Source: CAD feature listing. Evaluate the final solid. Frame: model axes, mm. Give positions to 0.01 mm unless a question says otherwise; leave off trailing zeros. Write each loop counter-clockwise with the first axis right and the second up, starting at its lowest first coordinate (ties: lowest second). Pieces come first, ordered by that corner, then holes. Notation, with made-up numbers: M 14,46.5 L 29,46.5 A34 ccw 29,80.5 Z; hole C 8,27.25 d4. An arc over 180 degrees is marked long. Answer as a JSON object with one key per item and string values. Group by question number.
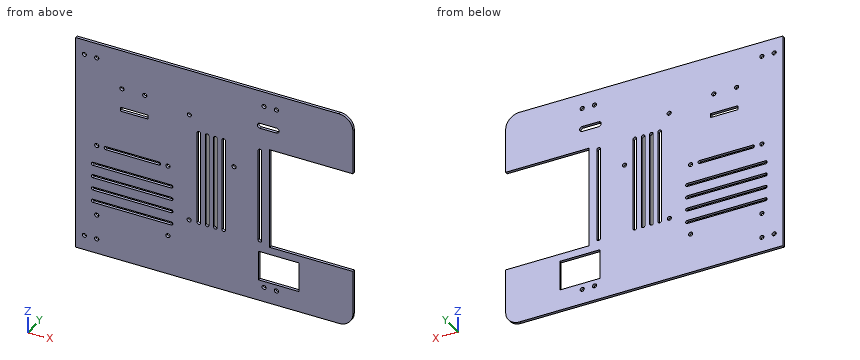
```python
from build123d import *

# Parameters (mm, degrees)
BOSS_EXTRUDE1_DEPTH = 2
SKETCH2_R           = 1.5
SKETCH2_W           = 19.920515559
SKETCH2_H           = 3.018311412
SKETCH2_W_2         = 29
SKETCH2_H_2         = 22
CUT_EXTRUDE1_DEPTH  = 2
FILLET1_R           = 10


with BuildPart() as part:
    # Sketch1 → Boss-Extrude1 (new body)
    with BuildSketch(Plane(origin=(0, 0, 0), x_dir=(1, 0, 0), z_dir=(0, 1, 0))):
        Polygon((62.5, -37.5), (62.5, -80.53), (-137.5, -80.53), (-137.5, 80.53), (62.5, 80.53), (62.5, 37.5), (2.5, 37.5), (2.5, -37.5), align=None)
    extrude(amount=BOSS_EXTRUDE1_DEPTH)

    # Sketch2 → Cut-Extrude1 (cut)
    with BuildSketch(Plane(origin=(0, 2, 0), x_dir=(1, 0, 0), z_dir=(0, 1, 0))):
        with Locations(Location((-131.256523302, -69.515826612, 0), (0, 0, 270))):
            Circle(SKETCH2_R)
        with Locations(Location((7.303150728, -69.515826612, 0), (0, 0, 270))):
            Circle(SKETCH2_R)
        with Locations(Location((-131.256523302, 69.515826612, 0), (0, 0, 90))):
            Circle(SKETCH2_R)
        with Locations(Location((7.303150728, 69.515826612, 0), (0, 0, 90))):
            Circle(SKETCH2_R)
        with Locations(Location((-122.332492344, -69.515826612, 0), (0, 0, 270))):
            Circle(SKETCH2_R)
        with Locations(Location((-1.623456056, -69.515826612, 0), (0, 0, 270))):
            Circle(SKETCH2_R)
        with Locations(Location((-1.623456056, 69.515826612, 0), (0, 0, 270))):
            Circle(SKETCH2_R)
        with Locations(Location((-122.332492344, 69.515826612, 0), (0, 0, 270))):
            Circle(SKETCH2_R)
        with Locations(Location((-23.238563778, -16.512077665, 0), (0, 0, 270))):
            Circle(SKETCH2_R)
        with Locations(Location((-55.491043914, -46.437145858, 0), (0, 0, 270))):
            Circle(SKETCH2_R)
        with Locations(Location((-55.618758711, 34.282977792, 0), (0, 0, 270))):
            Circle(SKETCH2_R)
        with Locations(Location((-70.912492344, 51.192828944, 0), (0, 0, 270))):
            Circle(SKETCH2_R)
        with Locations(Location((-122.332492344, 51.192828944, 0), (0, 0, 270))):
            Circle(SKETCH2_R)
        with Locations(Location((-122.332492344, -2.227171201, 0), (0, 0, 270))):
            Circle(SKETCH2_R)
        with Locations(Location((-70.912492344, -2.227171201, 0), (0, 0, 270))):
            Circle(SKETCH2_R)
        with Locations(Location((-104.14455224, -51.392693568, 0), (0, 0, 270))):
            Circle(SKETCH2_R)
        with Locations(Location((-87.673175627, -51.392693568, 0), (0, 0, 270))):
            Circle(SKETCH2_R)
        with BuildLine():
            Line((-3.265151958, 34.282977792), (-3.265151958, -34.42226179))
            ThreePointArc((-3.265151958, -34.42226179), (-4.562464061, -35.719573893), (-5.859776165, -34.42226179))
            Line((-5.859776165, -34.42226179), (-5.859776165, 34.282977792))
            ThreePointArc((-5.859776165, 34.282977792), (-4.562464061, 35.580289895), (-3.265151958, 34.282977792))
        make_face()
        with BuildLine():
            Line((-29.373558034, 34.282977792), (-29.373558034, -34.42226179))
            ThreePointArc((-29.373558034, -34.42226179), (-30.670870138, -35.719573893), (-31.968182241, -34.42226179))
            Line((-31.968182241, -34.42226179), (-31.968182241, 34.282977792))
            ThreePointArc((-31.968182241, 34.282977792), (-30.670870138, 35.580289895), (-29.373558034, 34.282977792))
        make_face()
        with BuildLine():
            Line((-35.373558034, 34.282977792), (-35.373558034, -34.42226179))
            ThreePointArc((-35.373558034, -34.42226179), (-36.670870138, -35.719573893), (-37.968182241, -34.42226179))
            Line((-37.968182241, -34.42226179), (-37.968182241, 34.282977792))
            ThreePointArc((-37.968182241, 34.282977792), (-36.670870138, 35.580289895), (-35.373558034, 34.282977792))
        make_face()
        with BuildLine():
            Line((-41.373558034, 34.282977792), (-41.373558034, -34.42226179))
            ThreePointArc((-41.373558034, -34.42226179), (-42.670870138, -35.719573893), (-43.968182241, -34.42226179))
            Line((-43.968182241, -34.42226179), (-43.968182241, 34.282977792))
            ThreePointArc((-43.968182241, 34.282977792), (-42.670870138, 35.580289895), (-41.373558034, 34.282977792))
        make_face()
        with BuildLine():
            Line((-47.373558034, 34.282977792), (-47.373558034, -34.42226179))
            ThreePointArc((-47.373558034, -34.42226179), (-48.670870138, -35.719573893), (-49.968182241, -34.42226179))
            Line((-49.968182241, -34.42226179), (-49.968182241, 34.282977792))
            ThreePointArc((-49.968182241, 34.282977792), (-48.670870138, 35.580289895), (-47.373558034, 34.282977792))
        make_face()
        with BuildLine():
            Line((-115.769074494, -1.056435162), (-77.456824006, -1.056435162))
            ThreePointArc((-77.456824006, -1.056435162), (-76.286087967, -2.227171201), (-77.456824006, -3.39790724))
            Line((-77.456824006, -3.39790724), (-115.769074494, -3.39790724))
            ThreePointArc((-115.769074494, -3.39790724), (-116.939810532, -2.227171201), (-115.769074494, -1.056435162))
        make_face()
        with Locations((-95.335675627, -35.460717912)):
            Rectangle(SKETCH2_W, SKETCH2_H)
        with BuildLine():
            Line((-68.521094286, 39.924878234), (-125.034135879, 39.924878234))
            ThreePointArc((-125.034135879, 39.924878234), (-126.207275741, 41.098018096), (-125.034135879, 42.271157959))
            Line((-125.034135879, 42.271157959), (-68.521094286, 42.271157959))
            ThreePointArc((-68.521094286, 42.271157959), (-67.347954424, 41.098018096), (-68.521094286, 39.924878234))
        make_face()
        with BuildLine():
            Line((-68.521094286, 30.449255701), (-125.034135879, 30.449255701))
            ThreePointArc((-125.034135879, 30.449255701), (-126.207275741, 31.622395563), (-125.034135879, 32.795535426))
            Line((-125.034135879, 32.795535426), (-68.521094286, 32.795535426))
            ThreePointArc((-68.521094286, 32.795535426), (-67.347954424, 31.622395563), (-68.521094286, 30.449255701))
        make_face()
        with BuildLine():
            Line((-68.521094286, 20.973633168), (-125.034135879, 20.973633168))
            ThreePointArc((-125.034135879, 20.973633168), (-126.207275741, 22.14677303), (-125.034135879, 23.319912892))
            Line((-125.034135879, 23.319912892), (-68.521094286, 23.319912892))
            ThreePointArc((-68.521094286, 23.319912892), (-67.347954424, 22.14677303), (-68.521094286, 20.973633168))
        make_face()
        with BuildLine():
            Line((-68.521094286, 11.498010634), (-125.034135879, 11.498010634))
            ThreePointArc((-125.034135879, 11.498010634), (-126.207275741, 12.671150497), (-125.034135879, 13.844290359))
            Line((-125.034135879, 13.844290359), (-68.521094286, 13.844290359))
            ThreePointArc((-68.521094286, 13.844290359), (-67.347954424, 12.671150497), (-68.521094286, 11.498010634))
        make_face()
        with Locations((8.983260953, 53.984235798)):
            Rectangle(SKETCH2_W_2, SKETCH2_H_2)
        with BuildLine():
            Line((7.303150728, -51.824271767), (-4.562464061, -51.824271767))
            ThreePointArc((-4.562464061, -51.824271767), (-6.461969906, -53.723777612), (-4.562464061, -55.623283456))
            Line((-4.562464061, -55.623283456), (7.303150728, -55.623283456))
            ThreePointArc((7.303150728, -55.623283456), (9.202656572, -53.723777612), (7.303150728, -51.824271767))
        make_face()
    extrude(amount=-CUT_EXTRUDE1_DEPTH, mode=Mode.SUBTRACT)

    # Fillet1
    fillet1_edges = [part.edges().sort_by_distance(p)[0] for p in [
        (62.5, 1, -80.53),
        (62.5, 1, 80.53),
    ]]
    fillet(fillet1_edges, radius=FILLET1_R)


solid = part.part
```
(1) Section D-D, the plane x = -98.5. Return loops of the section in (y, z), plus the area to 3 significant figures.
(2) Section B-B, the plane z = -4. Return loops of the section in (x, y), plus the area to 3 significant figures.
(3) Ray query, L1, parallel to X at y = 0.15, z = -26.5; L2, parallel to Z at x = 2, y = 0.2; L3, parallel to Z at x = 43, y = 0.2. Return the intervals inside material, ascending. Write a range as [from, to].
(4) Section C-C, the plane z = -62.5. Return loops of the section in (x, y), plus the area to 3 significant figures.
(5) Section A-A, the plane x = 37. Return loops of the section in (y, z), plus the area to 3 significant figures.
(6) Contact query for flat-ended pins moving along their axis: pin 1 Ø2.5 at (x, z) = (7.3, 69.52) entering from +Y; pin 2 Ø1 at (y, z) = (0.5, 8) entering from +X. Output: stop coordinate, or through.
Reported:
{
 "1": {"outline": "M 0,-80.53 L 2,-80.53 L 2,-42.27 L 0,-42.27 Z; M 0,-39.92 L 2,-39.92 L 2,-32.8 L 0,-32.8 Z; M 0,-30.45 L 2,-30.45 L 2,-23.32 L 0,-23.32 Z; M 0,-20.97 L 2,-20.97 L 2,-13.84 L 0,-13.84 Z; M 0,-11.5 L 2,-11.5 L 2,1.06 L 0,1.06 Z; M 0,3.4 L 2,3.4 L 2,33.95 L 0,33.95 Z; M 0,36.97 L 2,36.97 L 2,80.53 L 0,80.53 Z", "area": "293 mm2"},
 "2": {"outline": "M -137.5,0 L -49.97,0 L -49.97,2 L -137.5,2 Z; M -47.37,0 L -43.97,0 L -43.97,2 L -47.37,2 Z; M -41.37,0 L -37.97,0 L -37.97,2 L -41.37,2 Z; M -35.37,0 L -31.97,0 L -31.97,2 L -35.37,2 Z; M -29.37,0 L -5.86,0 L -5.86,2 L -29.37,2 Z; M -3.27,0 L 2.5,0 L 2.5,2 L -3.27,2 Z", "area": "254 mm2"},
 "3": {"L1": "x = [-137.5, -49.97], [-47.37, -43.97], [-41.37, -37.97], [-35.37, -31.97], [-29.37, -5.86], [-3.27, 2.5]", "L2": "z = [-80.53, -64.98], [-42.98, 51.82], [55.62, 80.53]", "L3": "z = [-80.53, -37.5], [37.5, 80.53]"},
 "4": {"outline": "M -137.5,0 L -5.52,0 L -5.52,2 L -137.5,2 Z; M 23.48,0 L 62.5,0 L 62.5,2 L 23.48,2 Z", "area": "342 mm2"},
 "5": {"outline": "M 0,-80.53 L 2,-80.53 L 2,-37.5 L 0,-37.5 Z; M 0,37.5 L 2,37.5 L 2,80.53 L 0,80.53 Z", "area": "172 mm2"},
 "6": {"pin 1": "passes through", "pin 2": "stops at x = 2.5"}
}
